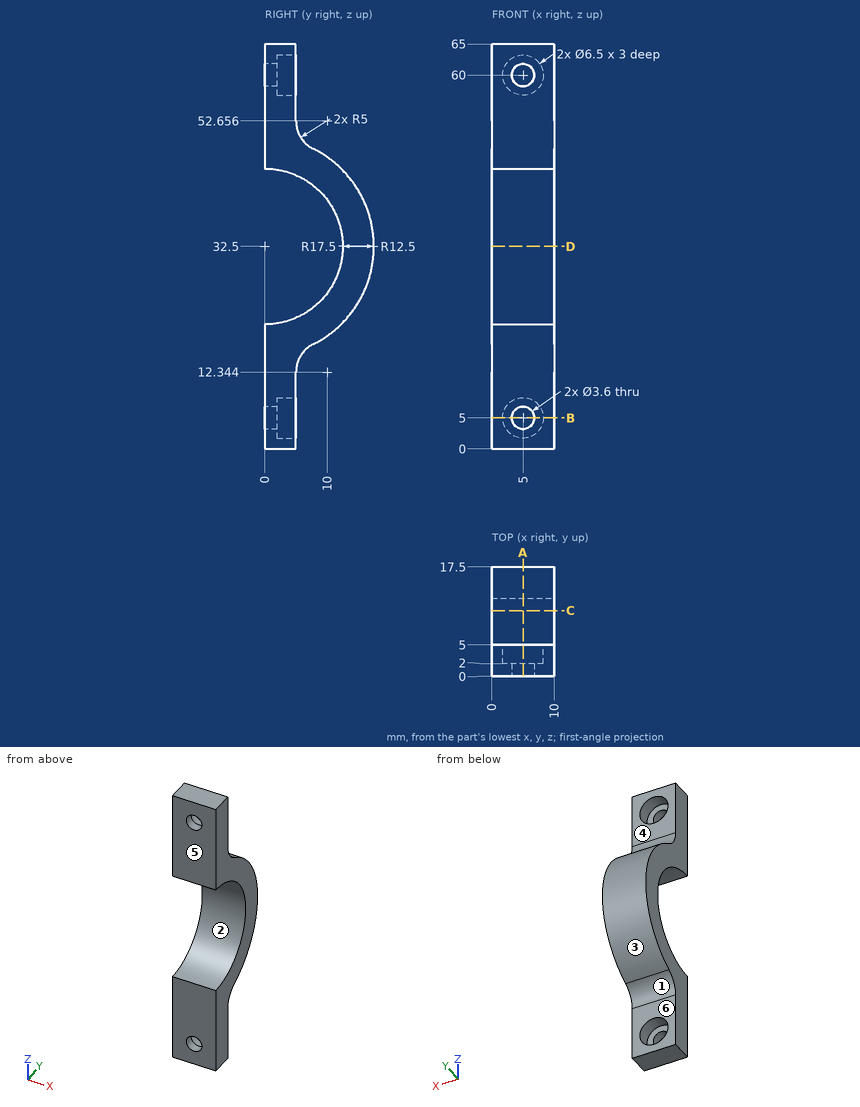
Print and shaded views of the part. All mm, measured from the part's lowest x, y and z. A direction names the side the tool comes from. Round coordinates to 2 decimals unless told otherwise and drop trailing zeros. Write each loop counter-clockwise with the first axis right and the second up, starting at its lowest first coordinate (ties: lowest second). Pieces come first, ordered by that corner, then holes. Notation, with made-up numbers: (16, -34.75) -> (73, -34.75) arc R19 ccw to (73, -12.75) -> close; hole circle Ø2 at (-35, 31). An arc over 180 degrees is marked (long way). Return JSON: item names as keys, results as strings. Group by question number.
Q1. Mould opens along Z. For the marked faces 1, 2, 3 and 4 say: pulls with the +Z half, pulls with the -Z half, needs draft (parallel to the pull), parting line crosses it, or undercut.
Q2. Saw through at C-C on y = 10.5. Write the cut outline in (x, z).
Q3. Saw through at D-D on z = 32.5. Write the cut outline in (x, y), plus the area to 3 significant figures.
Q4. Probe L1, parallel to Z at x = 5, y = 0.55; L2, parallel to X at y = 0.95, z = 60; L3, parallel to X at y = 3.4, z = 60. List the from-to ranges inside material, lowest first. Write a range as [from, to].
Q5. Saw through at B-B on z = 5. Write the cut outline in (x, y), plus the area to 3 significant figures.
Q6. Which spindle directions (+Z, -Z, +X, -X, +Y, -Y) get a long thin tool onto all of the face, cutting with end or side? Do the marked faces 5 and 6. Say none if no direction does.
Q7. Saw through at A-A on x = 5. State how many separate pieces and enclosed holes the cut face has.
Q8. Pin check, flat tips, straight feed: pin 1 (5 mm diameter, centred on x = 5, z = 4.5, fed in from +Y); pin 2 (3 mm diameter, centred on x = 2, z = 23, fed in from -Y) (1 decimal); pin 3 (3 mm diameter, centred on x = 4, z = 57, fed in from +Y); pin 4 (2 mm diameter, centred on x = 5, z = 60, fed in from -Y). Stop position of each tip, or through.
Answer:
{
 "1": {"face 1": "pulls with the -Z half", "face 2": "undercut", "face 3": "parting line crosses it", "face 4": "needs draft"},
 "2": {"outline": "(0, 18.5) -> (10, 18.5) -> (10, 25.72) -> (0, 25.72) -> close; (0, 39.28) -> (10, 39.28) -> (10, 46.5) -> (0, 46.5) -> close"},
 "3": {"outline": "(0, 12.5) -> (10, 12.5) -> (10, 17.5) -> (0, 17.5) -> close", "area": "50.0 mm2"},
 "4": {"L1": "[0, 3.2], [6.8, 20.01], [44.99, 58.2], [61.8, 65]", "L2": "[0, 3.2], [6.8, 10]", "L3": "[0, 1.75], [8.25, 10]"},
 "5": {"outline": "(0, 0) -> (3.2, 0) -> (3.2, 2) -> (1.75, 2) -> (1.75, 5) -> (0, 5) -> close; (6.8, 0) -> (10, 0) -> (10, 5) -> (8.25, 5) -> (8.25, 2) -> (6.8, 2) -> close", "area": "23.3 mm2"},
 "6": {"face 5": "+Z, -Z, +X, -X, -Y", "face 6": "-Z, +X, -X, +Y"},
 "7": {"separate pieces": "3", "enclosed holes": "0"},
 "8": {"pin 1": "y = 2", "pin 2": "y = 5.9", "pin 3": "y = 5", "pin 4": "through"}
}
